```python
from build123d import *

# Parameters (mm, degrees)
SKETCH1_R           = 2.75
BOSS_EXTRUDE1_DEPTH = 2
SKETCH2_R           = 4
SKETCH2_R_2         = 2.75
BOSS_EXTRUDE2_DEPTH = 4


with BuildPart() as part:
    # Sketch1 → Boss-Extrude1 (new body)
    with BuildSketch(Plane(origin=(0, 0, 0), x_dir=(0, 0, -1), z_dir=(1, 0, 0))):
        with BuildLine():
            Line((4, 0), (29, 0))
            ThreePointArc((29, 0), (33, 4), (29, 8))
            Line((29, 8), (4, 8))
            ThreePointArc((4, 8), (0, 4), (4, 0))
        make_face()
        with Locations((4, 4)):
            Circle(SKETCH1_R, mode=Mode.SUBTRACT)
        with Locations((29, 4)):
            Circle(SKETCH1_R, mode=Mode.SUBTRACT)
    extrude(amount=BOSS_EXTRUDE1_DEPTH)

    # Sketch2 → Boss-Extrude2 (add)
    with BuildSketch(Plane(origin=(0, 0, 0), x_dir=(0, 0, -1), z_dir=(1, 0, 0))):
        with Locations(Location((4, 4, 0), (0, 0, 270))):
            Circle(SKETCH2_R)
        with Locations((4, 4)):
            Circle(SKETCH2_R_2, mode=Mode.SUBTRACT)
    extrude(amount=BOSS_EXTRUDE2_DEPTH)


solid = part.part
```
The listing builds one solid part. Answer for the finished solid, in the listing's coordinates (mm). Round coordinates to 2 decimals unless told otherwise and drop trailing zeros. Order: outer loops, then holes, each group sorted by start corner. A loop starts at its lowest first (then second) coordinate and runs counter-clockwise, first axis right, second up. Notation, with made-up numbers: (46.5, 54.5) -> (62.5, 54.5) arc R10 cw to (62.5, 62.5) -> close; hole circle Ø1 at (-25, 79.25). An arc over 180 degrees is marked (long way). Answer as CSV lines item,"result". Start each with the question number.
(1) For a pull along Y with two mould halves and no side action, classify faces 1 (the face through (1, 4, -33)), 2 (the face through (0.986, 4.121, -26.253)), 3 (the face through (0, 4, -16)) as +Y half, -Y half, draft (parallel to the pull), parting line (faces both ways), or undercut.
(2) The part is cut by section B-B (x = 2.9). Determine the outline of the cut face in (y, z), then the cut area to 3 significant figures.
(3) The part is cut by section C-C (z = -11). Determine the outline of the cut face in (x, y), then the cut area to 3 significant figures.
(4) The part is cut by section D-D (x = 1.65). Determine the outline of the cut face in (y, z), then the cut area to 3 significant figures.
(5) Flat-ended cylindrical pins translate along their axes: pin 1 Ø2 at (y, z) = (3, -13.5) entering from +X; pin 2 Ø1.5 at (x, y) = (0.5, 5) entering from +Z. Find the tip coordinate at first contact, or state that the pin passes through.
(6) The part is cut by section A-A (y = 4). Determine the outline of the cut face in (x, z).
(7) Find the intervals of material crossed by probe 1 along Y at (x, z) = (0.6, -29); probe 2 along Z at (x, y) = (1.1, 4.25); probe 3 along Z at (x, y) = (1.1, 4.75), in increasing order. Write a range as from..to.
Evaluation:
1,face 1,"parting line"
1,face 2,"undercut"
1,face 3,"draft"
2,outline,"circle Ø8 at (4, -4); hole circle Ø5.5 at (4, -4)"
2,area,"26.5 mm²"
3,outline,"(0, 0) -> (2, 0) -> (2, 8) -> (0, 8) -> close"
3,area,"16.0 mm²"
4,outline,"(0, -29) arc R4 ccw to (8, -29) -> (8, -4) arc R4 ccw to (0, -4) -> close; hole circle Ø5.5 at (4, -29); hole circle Ø5.5 at (4, -4)"
4,area,"203 mm²"
5,pin 1,"x = 2"
5,pin 2,"z = -0.01"
6,outline,"(0, -33) -> (2, -33) -> (2, -31.75) -> (0, -31.75) -> close; (0, -26.25) -> (2, -26.25) -> (2, -8) -> (4, -8) -> (4, -6.75) -> (0, -6.75) -> close; (0, -1.25) -> (4, -1.25) -> (4, 0) -> (0, 0) -> close"
7,probe 1,"0..1.25, 6.75..8"
7,probe 2,"-32.99..-31.74, -26.26..-6.74, -1.26..-0.01"
7,probe 3,"-32.93..-31.65, -26.35..-6.65, -1.35..-0.07"
